Geometry: final body of the model. Coordinates: model frame, mm. A direction names the side the tool comes from. Round coordinates to 2 decimals unless told otherwise and drop trailing zeros. Loops run counter-clockwise (first coordinate to the right, second up) from the corner with the lowest first, then second, coordinate; pieces in that order, holes last. Notation, with made-up numbers: (-15.5, 23) - (4.5, 23) arc R33 cw to (4.5, 57) - close; hole circle Ø1 at (52.5, 39.5). An arc over 180 degrees is marked (long way). Write item = value, one per line. Start each with the question number.
Item 1: Line query: line 1 (X direction, y = 198, z = 1455); line 2 (Z direction, x = 327, y = -35); line 3 (Z direction, x = 160, y = 96). Output: solid intervals per line, ascending. Write a range as from..to.
Item 2: Access query for faces 4 (the flat face through (203.2, -5, 1386)), 5 (the flat face through (254, -5, 1357)), 6 (the flat face through (-254, -5, 1357)), 7 (the flat face through (-1, 76.2, 627)), 8 (the flat face through (-1, -76.2, 627)). Directions: +Z, -Z, +X, -X, +Y, -Y. A direction counts if a zero-diameter tool reaches every point of the face in a straight line with its end or side. Return the directions, or none.
Item 3: First-contact query: pin 1 (1 mm diameter, centred on y = 11.5, z = 738, fed in from -X). Flat tip, straight axial feed; report the tip coordinate or a pass-through.
Item 4: Draft query along X for faces 1 (the flat face through (76.2, 1, 627)), 2 (the flat face through (-4, 355.6, 1268)), 3 (the flat face through (-203.2, -5, 1386)). Return one class per face: pulls with the +X half, pulls with the -X half, needs draft (parallel to the pull), parting line crosses it, or undercut.
Item 5: Section A-A (z = 1430). Return loops of the section in (x, y).
Item 6: Section B-B (x = 101.5). Return loops of the section in (y, z), plus the area to 3 significant figures.
from build123d import *

# Parameters (mm, degrees)
F0_W     = 914.4
F0_H     = 914.4
F1_DEPTH = 50.8
F2_W     = 152.4
F2_H     = 152.4
F3_DEPTH = 1219.2
F4_W     = 508
F4_H     = 711.2
F5_DEPTH = 304.8
F6_W     = 406.4
F6_H     = 812.8
F7_DEPTH = 254
F8_R     = 25.39999


# Not quite as in the source:
# - a fillet or chamfer is up to 0.001 mm smaller than in the source, because OpenCascade refuses the exact size
# - a feature names something its author has since deleted; it is built from what else it names


with BuildPart() as f1:
    # F0 (on Top) → F1 (new body)
    with BuildSketch(Plane.XY):
        with Locations((11.3640455229, 0)):
            Rectangle(F0_W, F0_H)
    extrude(amount=F1_DEPTH)

    # F2 (on face) → F3 (join)
    with BuildSketch(Plane(origin=(0, 0, 0), x_dir=(1, 0, 0), z_dir=(0, 0, -1))):
        Rectangle(F2_W, F2_H)
    extrude(amount=-F3_DEPTH)

    # F4 (on face) → F5 (join)
    with BuildSketch(Plane.XY.offset(1219.2)):
        Rectangle(F4_W, F4_H)
    extrude(amount=F5_DEPTH)

    # F6 (on face) → F7 (cut)
    with BuildSketch(Plane.XY.offset(1524)):
        Rectangle(F6_W, F6_H)
    extrude(amount=-F7_DEPTH, mode=Mode.SUBTRACT)

    # F8 (radius 25.4 in the source; OpenCascade refuses exactly that, so slightly less here)
    f8_edges = [f1.edges().sort_by_distance(p)[0] for p in [
        (-254, 0, 1524),
        (-203.2, 0, 1524),
        (203.2, 0, 1524),
        (254, 0, 1524),
    ]]
    fillet(f8_edges, radius=F8_R)


solid = f1.part
Taken from the geometry:
q1.line_1 = -254..-203.2, 203.2..254
q1.line_2 = 0..50.8
q1.line_3 = 0..50.8, 1219.2..1270
q2.face_4 = +Z, +Y, -Y
q2.face_5 = +Z, +X, +Y, -Y
q2.face_6 = +Z, -X, +Y, -Y
q2.face_7 = +X, -X, +Y
q2.face_8 = +X, -X, -Y
q3.pin_1 = -76.2
q4.face_1 = pulls with the +X half
q4.face_2 = needs draft
q4.face_3 = undercut
q5.outline = (-254, -355.6) - (-203.2, -355.6) - (-203.2, 355.6) - (-254, 355.6) - close; (203.2, -355.6) - (254, -355.6) - (254, 355.6) - (203.2, 355.6) - close
q6.outline = (-457.2, 0) - (457.2, 0) - (457.2, 50.8) - (-457.2, 50.8) - close; (-355.6, 1219.2) - (355.6, 1219.2) - (355.6, 1270) - (-355.6, 1270) - close
q6.area = 82,600 mm^2
